Autodesk Inventor part; units mm, degrees
ref_plane "nut_XY" through (6, 0, 0) normal (1, 0, 0) x (0, 0, -1)
ref_plane "nut_YZ" through (6, 0, 0) normal (0, 0, -1) x (0, 1, 0)
ref_plane "nut_ZX" through (6, 0, 0) normal (0, 1, 0) x (1, 0, 0)
sketch "Sketch_1" plane through (0, 0, 0) normal (0, 0, 1) x (1, 0, 0)
  line L0 (6, 0) -> (-3, 0)
  line L1 (-3, 0) -> (-3, 2.45)
  line L2 (-3, 2.45) -> (-2.7, 2.75)
  line L3 (-2.7, 2.75) -> (0, 2.75)
  line L4 (0, 2.75) -> (0, 1.5)
  line L5 (0, 1.5) -> (5.6935, 1.5)
  line L6 (5.6935, 1.5) -> (6, 1.1935)
  line L7 (6, 1.1935) -> (6, 0)
  line L8 (6, 0) -> (-3, 0)
revolve "Revolution1" add sketch "Sketch_1" angle 360 about axis through (6, 0, 0) along (1, 0, 0)
thread "Thread1"
sketch "Sketch_4" plane through (0, 0, 0) normal (0, 0, 1) x (1, 0, 0)
  line L0 (-1.1651, 0) -> (-3, 0)
  line L1 (-3, 0) -> (-3, 1.25)
  line L2 (-3, 1.25) -> (-1.5, 1.25)
  line L3 (-1.5, 1.25) -> (-1.1651, 0)
  line L4 (-1.1651, 0) -> (-3, 0)
revolve "Revolution2" cut sketch "Sketch_4" angle 360 about axis through (-1.1651, 0, 0) along (1, 0, 0)
sketch "Sketch_3" plane through (-3, 0, 0) normal (1, 0, 0) x (0, 0, -1)
  line L0 (-1.25, 0.7217) -> (-1.25, -0.7217)
  line L1 (-1.25, -0.7217) -> (0, -1.4434)
  line L2 (0, -1.4434) -> (1.25, -0.7217)
  line L3 (1.25, -0.7217) -> (1.25, 0.7217)
  line L4 (1.25, 0.7217) -> (0, 1.4434)
  line L5 (0, 1.4434) -> (-1.25, 0.7217)
extrude "Extrusion1" cut sketch "Sketch_3" along normal blind 1.5
ref_plane "nut_XY" through (6, 0, 0) normal (1, 0, 0) x (0, 0, -1)
ref_plane "nut_YZ" through (6, 0, 0) normal (0, 0, -1) x (0, 1, 0)
ref_plane "nut_ZX" through (6, 0, 0) normal (0, 1, 0) x (1, 0, 0)
ref_plane "bolt_XY" through (0, 0, 0) normal (1, 0, 0) x (0, 0, -1)
ref_plane "bolt_YZ" through (0, 0, 0) normal (0, 0, -1) x (0, 1, 0)
ref_plane "bolt_ZX" through (0, 0, 0) normal (0, 1, 0) x (1, 0, 0)
properties part number "SCB3-6_1"
The model under review builds one solid part; all positions refer to its coordinate system, in mm. A direction names the side the tool comes from. Round coordinates to 2 decimals unless told otherwise and drop trailing zeros. Order: outer loops, then holes, each group sorted by start corner. A loop starts at its lowest first (then second) coordinate and runs counter-clockwise, first axis right, second up.
(1) Tool access review of faces 5 (the face through (-2, 0, -1.25)), 6 (the face through (-3, 1.1, -1.1)), 7 (the face through (2.89, -1.5, 0.07)): name each direction out of +Z, -Z, +X, -X, +Y, -Y from which nothing blocks a thin tool from reaching the whole face with its end or side.
Working result:
face 5: -X
face 6: +Z, -Z, -X, +Y, -Y
face 7: +X
(2) Mouldability with a two-part tool opening along Z and no side actions: class faces 1 (the face through (-2.26, -1.08, 0.63)), 2 (the face through (-2.26, 1.088, 0.616)), 3 (the face through (-1.331, -0.596, -2.685)), 4 (the face through (0, 1.2, -1.2)) as released by +Z, released by -Z, zero draft, split by the parting line, or undercut.
Working result:
face 1: undercut
face 2: undercut
face 3: split by the parting line
face 4: zero draft
(3) Take a section at A-A, the plane x = -2. State the section outline as (y, z) points.
Working result:
outline: circle Ø5.5 at (0, 0); hole (-1.44, 0) - (-0.72, -1.25) - (0.72, -1.25) - (1.44, 0) - (0.72, 1.25) - (-0.72, 1.25) - close
(4) For P1, Ø1, axis at x = -1.5, z = 2, coming from the +Y side; P2, Ø2, axis at y = -2, z = 2, coming from the +X side; P3, Ø1, axis at x = -1, y = 1.5, coming from the -Z side, all flat-tipped, find the tip position at first contact; note any pin that passes through.
Working result:
P1: stops at y = 2.3
P2: stops at x = 0
P3: stops at z = -2.56
(5) Take a section at B-B, the plane x = 3.75. State the section outline as (y, z) points, plus the area to 3 significant figures.
Working result:
outline: circle Ø3 at (0, 0)
area: 7.07 mm2
(6) Wall thickness on L1, parallel to X at y = 1.65, z = -1.8; L2, parallel to Z at x = 1.25, y = -1; L3, parallel to X at y = -0.65, z = -0.2: over which ranges is each line inside the solid? List them lowest first.
Working result:
L1: x = -3 to 0
L2: z = -1.12 to 1.12
L3: x = -1.35 to 6
